```python
from build123d import *

# Parameters (mm, degrees)
F0_R     = 8.73125
F1_DEPTH = 6.35
F2_R     = 2.032
F3_DEPTH = 25.4
F4_SIZE  = 0.508


with BuildPart() as f1:
    # F0 (on Top) → F1 (new body)
    with BuildSketch(Plane.XY):
        Circle(F0_R)
    extrude(amount=F1_DEPTH)

    # F2 (on face) → F3 (cut)
    with BuildSketch(Plane.XY.offset(6.35)):
        Circle(F2_R)
    extrude(amount=-F3_DEPTH, mode=Mode.SUBTRACT)

    # F4
    f4_edges = [f1.edges().sort_by_distance(p)[0] for p in [
        (-8.73125, 0, 0),
        (-8.73125, 0, 6.35),
        (-2.032, 0, 6.35),
        (-2.032, 0, 0),
    ]]
    chamfer(f4_edges, length=F4_SIZE)


solid = f1.part
```
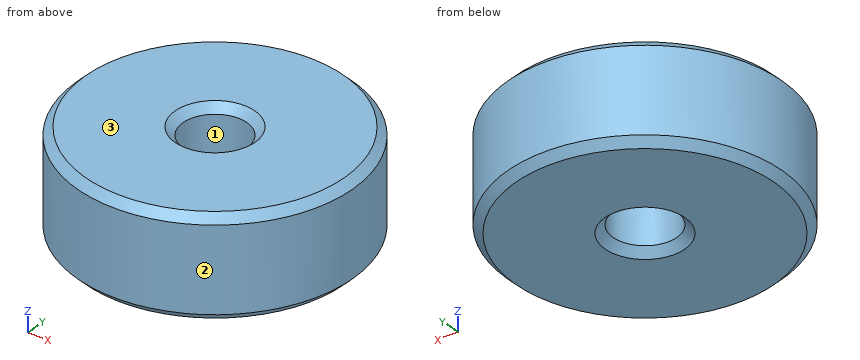
Geometry check sheet. Reference: the model listing, model coordinates, mm. Face numbers are marked on the shaded views. Round coordinates to 2 decimals unless told otherwise and drop trailing zeros. Order: outer loops, then holes, each group sorted by start corner. A loop starts at its lowest first (then second) coordinate and runs counter-clockwise, first axis right, second up. Notation, with made-up numbers: (55.5, -3) - (72.5, -3) arc R19 cw to (72.5, 9) - close; hole circle Ø10 at (5.5, -9). An arc over 180 degrees is marked (long way). Use a Markdown table: item, result. Add a question column.
(1) Sectioned sample at A-A, the plane y = 0. Enter the section's corners in (x, z), and give its area (3 significant figures).
(2) Material ranges on line 1 along Y through (x, z) = (0, 4.5); line 2 along X through (y, z) = (0.5, 3.25); line 3 along Y through (x, z) = (-7.75, 4.5), recorded low to high. Write a range as [from, to].
(3) Depth check by flat-ended pin: pin 1 (1 mm diameter, centred on x = 3.5, z = 2.5, fed in from +Y); pin 2 (5.5 mm diameter, centred on x = 0, y = 0, fed in from -Z); pin 3 (2 mm diameter, centred on x = -7, z = 1.5, fed in from +Y); pin 4 (2 mm diameter, centred on y = 5.5, z = 5.5, fed in from -X). Enter the tip coordinate at first touch or a pass-through.
(4) Release check for a two-part mould opening along Y. For the marked faces 1, 2 and 3 record: pulls with the +Y half, pulls with the -Y half, needs draft (parallel to the pull), parting line crosses it, or undercut.
(5) Sectioned sample at C-C, the plane z = 4. Enter the section's corners in (x, y), and give its area (3 significant figures).
Answers below:
| question | item | result |
|---|---|---|
| 1 | outline | (-8.73, 0.51) - (-8.22, 0) - (-2.54, 0) - (-2.03, 0.51) - (-2.03, 5.84) - (-2.54, 6.35) - (-8.22, 6.35) - (-8.73, 5.84) - close; (2.03, 0.51) - (2.54, 0) - (8.22, 0) - (8.73, 0.51) - (8.73, 5.84) - (8.22, 6.35) - (2.54, 6.35) - (2.03, 5.84) - close |
| 1 | area | 84.0 mm² |
| 2 | line 1 | [-8.73, -2.03], [2.03, 8.73] |
| 2 | line 2 | [-8.72, -1.97], [1.97, 8.72] |
| 2 | line 3 | [-4.02, 4.02] |
| 3 | pin 1 | y = 8.2 |
| 3 | pin 2 | z = 0 |
| 3 | pin 3 | y = 6.34 |
| 3 | pin 4 | x = -7.48 |
| 4 | face 1 | undercut |
| 4 | face 2 | parting line crosses it |
| 4 | face 3 | needs draft |
| 5 | outline | circle Ø17.46 at (0, 0); hole circle Ø4.06 at (0, 0) |
| 5 | area | 227 mm² |
